from build123d import *

# Parameters (mm, degrees)
SKETCH1_R           = 23.31
BOSS_EXTRUDE1_DEPTH = 15
SKETCH2_R           = 23.31
BOSS_EXTRUDE2_DEPTH = 3
BOSS_EXTRUDE5_DEPTH = 134.3
SKETCH4_OUTSIDE_W   = 81.812
SKETCH4_OUTSIDE_H   = 81.812
SKETCH4_OUTSIDE_R   = 23.31
CUT_EXTRUDE2_DEPTH  = 204
SKETCH5_R           = 26.095
BOSS_EXTRUDE6_DEPTH = 3.35


with BuildPart() as part:
    # Sketch1 → Boss-Extrude1 (new body)
    with BuildSketch(Plane.XY):
        Circle(SKETCH1_R)
    extrude(amount=BOSS_EXTRUDE1_DEPTH)

    # Sketch2 → Boss-Extrude2 (add)
    with BuildSketch(Plane.XY.offset(15)):
        Circle(SKETCH2_R)
    extrude(amount=BOSS_EXTRUDE2_DEPTH)

    # Sketch3 → Boss-Extrude5 (add)
    with BuildSketch(Plane.XY.offset(18)):
        with BuildLine():
            Line((-19.00086471, 19.418454901), (-19.738244764, 18.741128654))
            Line((-19.738244764, 18.741128654), (-0.707086702, -0.005328765))
            Line((-0.707086702, -0.005328765), (-16.710421631, -16.2517048))
            ThreePointArc((-16.710421631, -16.2517048), (-16.44680571, -16.518434609), (-16.178932822, -16.780888914))
            Line((-16.178932822, -16.780888914), (-0.172775102, -0.531647218))
            Line((-0.172775102, -0.531647218), (20.92357267, -21.312399704))
            Line((20.92357267, -21.312399704), (21.625330607, -20.599984237))
            Line((21.625330607, -20.599984237), (0.528982835, 0.180768249))
            Line((0.528982835, 0.180768249), (16.535140556, 16.430009945))
            ThreePointArc((16.535140556, 16.430009945), (16.26867879, 16.693896801), (15.998006164, 16.953462737))
            Line((15.998006164, 16.953462737), (-0.005328765, 0.707086702))
            Line((-0.005328765, 0.707086702), (-19.00086471, 19.418454901))
        make_face()
    extrude(amount=BOSS_EXTRUDE5_DEPTH)

    # Sketch4 outside → Cut-Extrude2 (cut)
    with BuildSketch(Plane.XY.offset(18)):
        Rectangle(SKETCH4_OUTSIDE_W, SKETCH4_OUTSIDE_H)
        with Locations(Location((0, 0, 0), (0, 0, 136.660875724))):
            Circle(SKETCH4_OUTSIDE_R, mode=Mode.SUBTRACT)
    extrude(amount=CUT_EXTRUDE2_DEPTH, mode=Mode.SUBTRACT)

    # Sketch5 → Boss-Extrude6 (add)
    with BuildSketch(Plane.XY.offset(152.3)):
        Circle(SKETCH5_R)
    extrude(amount=BOSS_EXTRUDE6_DEPTH)


solid = part.part
Work out the finished part from the listing and answer in its coordinate system (mm). A direction names the side the tool comes from. Give positions to 0.01 mm unless a question says otherwise; leave off trailing zeros. Write each loop counter-clockwise with the first axis right and the second up, starting at its lowest first coordinate (ties: lowest second). Pieces come first, ordered by that corner, then holes.
Q1. The part is cut by section C-C on z = 44. Give the vertices of the cut face in (x, y).
Answer:
outline: (-16.95, 16) - (-0.71, -0.01) - (-16.71, -16.25) arc R23.31 ccw to (-16.18, -16.78) - (-0.17, -0.53) - (16.25, -16.71) arc R23.31 ccw to (16.95, -16) - (0.53, 0.18) - (16.54, 16.43) arc R23.31 ccw to (16, 16.95) - (-0.01, 0.71) - (-16.25, 16.71) arc R23.31 ccw to start
Q2. A tool of negligible diameter and unlimited length cuts with its end or side. For faces 4 (the face through (-15, 0, 18)), 5 (the face through (8.42, 8.19, 84.21)), 6 (the face through (0, 15, 18)), 7 (the face through (0, -5, 152.3)), 8 (the face through (7.924, -8.508, 84.21)), from which of +Z, -Z, +X, -X, +Y, -Y can it reach the whole face along a straight path? Write none if from no direction.
Answer:
face 4: -X
face 5: +X
face 6: +Y
face 7: none
face 8: -Y
Q3. Straight lines are drawn through the part: L1, parallel to Z at x = 1.5, y = -18; L2, parallel to Z at x = 17, y = -19.5; L3, parallel to Y at x = 3.5, z = 142. For each, find the intervals that lie inside material, in ascending order.
Answer:
L1: z = 0 to 18, 152.3 to 155.65
L2: z = 152.3 to 155.65
L3: y = -4.15 to -2.75, 3.2 to 4.27
Q4. The part is cut by section B-B on x = 13.5. Give the vertices of the cut face in (y, z).
Answer:
outline: (-22.33, 152.3) - (-14, 152.3) - (-14, 18) - (-19, 18) - (-19, 0) - (19, 0) - (19, 18) - (14.42, 18) - (14.42, 152.3) - (22.33, 152.3) - (22.33, 155.65) - (-22.33, 155.65) - close; hole (-12.6, 18) - (13.35, 18) - (13.35, 152.3) - (-12.6, 152.3) - close
Q5. The part is cut by section A-A on y = -5. Give the vertices of the cut face in (x, z).
Answer:
outline: (-25.61, 152.3) - (-5.63, 152.3) - (-5.63, 18) - (-22.77, 18) - (-22.77, 0) - (22.77, 0) - (22.77, 18) - (5.79, 18) - (5.79, 152.3) - (25.61, 152.3) - (25.61, 155.65) - (-25.61, 155.65) - close; hole (-4.57, 18) - (4.36, 18) - (4.36, 152.3) - (-4.57, 152.3) - close
Q6. For a pull along Y with two mould halves and no side action, classify faces 1 (the face through (-8.015, 8.597, 84.21)), 2 (the face through (0, -14, 18)), 3 (the face through (14, 0, 18)) as released by +Y, released by -Y, zero draft, split by the parting line, or undercut.
Answer:
face 1: released by +Y
face 2: zero draft
face 3: undercut
Q7. Given pin 1 (8 mm diameter, centred on y = 15.5, z = 41.5, fed in from -X); pin 2 (1.5 mm diameter, centred on y = -4.5, z = 97, fed in from +X); pin 3 (3 mm diameter, centred on x = -18, z = 28.5, fed in from +Y), each flat-ended and moving along its own axis, determine where each tip first touches the part or whether it passes through.
Answer:
pin 1: stops at x = -16.95
pin 2: stops at x = 6.04
pin 3: stops at y = 16.47
